Source: CAD feature listing. Evaluate the final solid. Frame: model axes, mm. A direction names the side the tool comes from. Coordinates: 2 decimals unless noted, no trailing zeros. Order: outer loops, then holes, each group sorted by start corner. A loop starts at its lowest first (then second) coordinate and runs counter-clockwise, first axis right, second up. Notation, with made-up numbers: (58.5, 52) -> (89.5, 52) arc R21 ccw to (89.5, 66) -> close; hole circle Ø11 at (-33.75, -25.75). An arc over 180 degrees is marked (long way). Write item = value, one per line. Start each with the question number.
Item 1: Section query C-C (y = -4.5). Output: boundary loops of the cut face in (x, z), then the cut area to 3 significant figures.
Item 2: Ray query, line 1 along X through (y, z) = (1, 5.08); line 2 along Y through (x, z) = (39.5, 28); line 3 along Y through (x, z) = (75, 42.5). Return the intervals inside material, ascending. Write a range as [from, to].
Item 3: Section query B-B (x = 123). Output: boundary loops of the cut face in (y, z).
Item 4: Set-up query: faces 5 (the cylindrical face through (32, 1, 4)), 6 (the flat face through (102.108, 4, 26)), 7 (the flat face through (99.568, 4, 26)). Return all of +Z, -Z, +X, -X, +Y, -Y with unobstructed straight access to the full face (end or side cutting, diameter ignored); none if empty.
Item 5: Contact query for flat-ended pins moving along their axis: pin 1 (3.5 mm diameter, centred on x = 102, z = 4.5, fed in from +Y); pin 2 (10 mm diameter, centred on x = 74.5, y = -11.5, fed in from -Z); pin 3 (6 mm diameter, centred on x = 50, z = 6, fed in from -Y). Output: stop coordinate, or through.
Item 6: Section query A-A (z = 5.08). Output: boundary loops of the cut face in (x, y).
Item 7: Mould query, pull axis X, two halves, no side actions, for faces 1 (the cylindrical face through (103.873, 1.288, 5.275)), 2 (the flat face through (133.35, -4, 27)), 3 (the cylindrical face through (19.625, 1.288, 4.388)), 4 (the flat face through (65.742, -7.714, 16.249)). Classes: released by +X, released by -X, zero draft, split by the parting line, or undercut.
Item 8: Section query D-D (z = 34.5). Output: boundary loops of the cut face in (x, y), then the cut area to 3 significant figures.
```python
from build123d import *

# Parameters (mm, degrees)
SKETCH1_W           = 133.35
SKETCH1_H           = 45.466
BOSS_EXTRUDE1_DEPTH = 2.54
CUT_EXTRUDE1_DEPTH  = 141.91072087
SKETCH4_W           = 2.54
SKETCH4_H           = 5.08
BOSS_EXTRUDE2_DEPTH = 4.572
SKETCH5_R           = 0.762
CUT_EXTRUDE2_DEPTH  = 112.999023942
FILLET1_R           = 2.54
FILLET2_R           = 2.54
FILLET3_R           = 1.27
BOSS_EXTRUDE4_DEPTH = 133.35
SKETCH10_R          = 1.4986
CUT_EXTRUDE3_DEPTH  = 2.54


with BuildPart() as part:
    # Sketch1 → Boss-Extrude1 (new body)
    with BuildSketch(Plane(origin=(0, 0, 0), x_dir=(1, 0, 0), z_dir=(0, 1, 0))):
        with Locations((66.675, -22.733)):
            Rectangle(SKETCH1_W, SKETCH1_H)
    extrude(amount=BOSS_EXTRUDE1_DEPTH)

    # Sketch2 → Cut-Extrude1 (cut, through all)
    with BuildSketch(Plane(origin=(133.35, 0, 0), x_dir=(0, 0, -1), z_dir=(1, 0, 0))):
        Polygon((-45.466, 0), (-45.466, 2.54), (-42.926, 2.54), align=None)
    extrude(amount=-CUT_EXTRUDE1_DEPTH, mode=Mode.SUBTRACT)

    # Sketch4 → Boss-Extrude2 (add)
    with BuildSketch(Plane(origin=(0, 2.54, 0), x_dir=(1, 0, 0), z_dir=(0, 1, 0))):
        with Locations((100.838, -25.4)):
            Rectangle(SKETCH4_W, SKETCH4_H)
    extrude(amount=BOSS_EXTRUDE2_DEPTH)

    # Sketch5 → Cut-Extrude2 (cut, through all)
    with BuildSketch(Plane(origin=(102.108, 0, 0), x_dir=(0, 0, -1), z_dir=(1, 0, 0))):
        with Locations((-25.4, 4.826)):
            Circle(SKETCH5_R)
    extrude(amount=-CUT_EXTRUDE2_DEPTH, mode=Mode.SUBTRACT)

    # Fillet1
    fillet1_edges = [part.edges().sort_by_distance(p)[0] for p in [
        (100.838, 7.112, 27.94),
    ]]
    fillet(fillet1_edges, radius=FILLET1_R)

    # Fillet2
    fillet2_edges = [part.edges().sort_by_distance(p)[0] for p in [
        (100.838, 7.112, 22.86),
    ]]
    fillet(fillet2_edges, radius=FILLET2_R - 0.0001)  # a hair under: the kernel refuses the full size

    # Fillet3
    fillet3_edges = [part.edges().sort_by_distance(p)[0] for p in [
        (66.675, 0, 0),
        (66.675, 2.54, 0),
    ]]
    fillet(fillet3_edges, radius=FILLET3_R - 0.0001)  # a hair under: the kernel refuses the full size

    # Sketch8 → Boss-Extrude4 (add)
    with BuildSketch(Plane.ZY):
        Polygon((1.27, -0.724150623), (31.652500271, -14.902671748), (45.466, 0), (1.27, 0), align=None)
        with BuildLine():
            ThreePointArc((0, 1.27), (0.344458941, 0.087889947), (1.27, -0.724150623))
            Line((1.27, -0.724150623), (1.27, 0))
            ThreePointArc((1.27, 0), (0.371974388, 0.371974388), (0, 1.27))
        make_face()
    extrude(amount=-BOSS_EXTRUDE4_DEPTH)

    # Sketch10 → Cut-Extrude3 (cut)
    with BuildSketch(Plane(origin=(0, 2.54, 0.507603591), x_dir=(1, 0, 0), z_dir=(0, -1, 0))):
        with Locations(Location((20.955, 4.572396409, 0), (0, 0, 270))):
            Circle(SKETCH10_R)
        with Locations(Location((30.9626, 4.572396409, 0), (0, 0, 270))):
            Circle(SKETCH10_R)
        with Locations(Location((102.3874, 4.572396409, 0), (0, 0, 270))):
            Circle(SKETCH10_R)
        with Locations(Location((112.395, 4.572396409, 0), (0, 0, 270))):
            Circle(SKETCH10_R)
    extrude(amount=CUT_EXTRUDE3_DEPTH, mode=Mode.SUBTRACT)


solid = part.part
```
Computed:
q1.outline = (0, 9.36) -> (133.35, 9.36) -> (133.35, 41.29) -> (0, 41.29) -> close
q1.area = 4,260 mm^2
q2.line_1 = [0, 19.46], [22.45, 29.46], [32.46, 100.89], [103.89, 110.9], [113.89, 133.35]
q2.line_2 = [-13.2, 2.54]
q2.line_3 = [-3.2, 2.54]
q3.outline = (-14.9, 31.65) -> (-0.72, 1.27) arc R2.2 ccw to (1.27, 0) arc R1.27 ccw to (2.54, 1.27) -> (2.54, 42.93) -> (0, 45.47) -> close
q4.face_5 = +Y
q4.face_6 = +Z, -Z, +X, +Y
q4.face_7 = +Z, -Z, -X, +Y
q5.pin_1 = 2.54
q5.pin_2 = 13.65
q5.pin_3 = -4.33
q6.outline = (0, -2.5) -> (133.35, -2.5) -> (133.35, 2.54) -> (113.89, 2.54) -> (113.89, 0) -> (110.9, 0) -> (110.9, 2.54) -> (103.89, 2.54) -> (103.89, 0) -> (100.89, 0) -> (100.89, 2.54) -> (32.46, 2.54) -> (32.46, 0) -> (29.46, 0) -> (29.46, 2.54) -> (22.45, 2.54) -> (22.45, 0) -> (19.46, 0) -> (19.46, 2.54) -> (0, 2.54) -> close
q7.face_1 = undercut
q7.face_2 = released by +X
q7.face_3 = undercut
q7.face_4 = zero draft
q8.outline = (0, -11.83) -> (133.35, -11.83) -> (133.35, 2.54) -> (0, 2.54) -> close
q8.area = 1,920 mm^2
